from build123d import *

# Parameters (mm, degrees)
PAD026_DEPTH      = 10
SKETCH046_R       = 1.6
POCKET018_DEPTH   = 15.001
SKETCH047_R       = 4
POCKET019_DEPTH   = 2
POCKET019_FACE6_W = 8
POCKET019_FACE6_H = 20
POCKET024_DEPTH   = 6.1
CHAMFER008_SIZE   = 2
FILLET014_R       = 10
FILLET015_R       = 3
CHAMFER009_SIZE   = 1
SKETCH048_R       = 2.1
POCKET020_DEPTH   = 15.4865555595
CHAMFER010_SIZE   = 0.6


with BuildPart() as part:
    # Sketch045 → Pad026 (new body, symmetric)
    with BuildSketch(Plane.XY):
        Polygon((40, 50), (45, 50), (45, 38.2679491924), (37.9807621135, 34.2153903092), (43.3012701892, 25), (48.6217782649, 15.7846096908), (41.6935750346, 11.7846096908), (36.3730669589, 21), (30, 32.0384757729), (30, 40), (40, 40), align=None)
    extrude(amount=PAD026_DEPTH, both=True)

    # Sketch046 (on Face5 of Pad026) → Pocket018 (cut, through all)
    with BuildSketch(Plane.YZ.offset(45)):
        with Locations((45, 0)):
            Circle(SKETCH046_R)
    extrude(amount=-POCKET018_DEPTH, mode=Mode.SUBTRACT)

    # Sketch047 (on Face9 of Pocket018) → Pocket019 (cut)
    with BuildSketch(Plane.YZ.offset(45)):
        with Locations((45, 0)):
            Circle(SKETCH047_R)
    extrude(amount=-POCKET019_DEPTH, mode=Mode.SUBTRACT)

    # Pocket019 Face6 → Pocket024 (cut)
    with BuildSketch(Plane(origin=(45.1576766498, 13.7846096908, 0), x_dir=(-0.8660254038, -0.5, 0), z_dir=(0.5, -0.8660254038, 0))):
        Rectangle(POCKET019_FACE6_W, POCKET019_FACE6_H)
    extrude(amount=-POCKET024_DEPTH, mode=Mode.SUBTRACT)

    # Chamfer008
    chamfer008_edges = [part.edges().sort_by_distance(p)[0] for p in [
        (42.5, 50, 10),
        (42.5, 50, -10),
        (42.107677, 19.067365, 10),
        (42.107677, 19.067365, -10),
    ]]
    chamfer(chamfer008_edges, length=CHAMFER008_SIZE)

    # Fillet014
    fillet014_edges = [part.edges().sort_by_distance(p)[0] for p in [
        (30, 32.038476, 0),
    ]]
    fillet(fillet014_edges, radius=FILLET014_R)

    # Fillet015
    fillet015_edges = [part.edges().sort_by_distance(p)[0] for p in [
        (45, 38.267949, 0),
    ]]
    fillet(fillet015_edges, radius=FILLET015_R)

    # Chamfer009
    chamfer009_edges = [part.edges().sort_by_distance(p)[0] for p in [
        (30, 40, 0),
    ]]
    chamfer(chamfer009_edges, length=CHAMFER009_SIZE)

    # Sketch048 (on Face13 of Chamfer009) → Pocket020 (cut, through all)
    with BuildSketch(Plane(origin=(43.3012701892, 25, 0), x_dir=(-0.5, 0.8660254038, 0), z_dir=(0.8660254038, 0.5, 0))):
        Circle(SKETCH048_R)
    extrude(amount=-POCKET020_DEPTH, mode=Mode.SUBTRACT)

    # Chamfer010
    chamfer010_edges = [part.edges().sort_by_distance(p)[0] for p in [
        (44.35127, 23.181347, 0),
        (37.423067, 19.181347, 0),
    ]]
    chamfer(chamfer010_edges, length=CHAMFER010_SIZE)


with BuildPart() as part_1:
    # Body026 placement: moved
    add(part.part.moved(Location((0, 0, 56))))


solid = part_1.part
Verification items for the finished model (mm, model axes). A direction names the side the tool comes from. Coordinates: 2 decimals unless noted, no trailing zeros. Order: outer loops, then holes, each group sorted by start corner. A loop starts at its lowest first (then second) coordinate and runs counter-clockwise, first axis right, second up.
Item 1: Material ranges on L1, parallel to Z at x = 42.15, y = 45; L2, parallel to Z at x = 44.55, y = 45; L3, parallel to Y at x = 40.25, z = 55, recorded low to high.
Filled in:
L1: z = 46 to 54.4, 57.6 to 66
L2: z = 46 to 52, 60 to 66
L3: y = 17.99 to 21.11, 25.37 to 30.28, 35.53 to 43.75, 46.25 to 50
Item 2: Depth check by flat-ended pin: pin 1 (2 mm diameter, centred on y = 38, z = 56.5, fed in from +X); pin 2 (4 mm diameter, centred on x = 40.5, z = 63, fed in from -Y); pin 3 (6.5 mm diameter, centred on y = 46.5, z = 57, fed in from +X); pin 4 (1.9 mm diameter, centred on y = 45, z = 56, fed in from -X). Enter the tip coordinate at first touch or a pass-through.
Filled in:
pin 1: stops at x = 44.83
pin 2: stops at y = 17.07
pin 3: stops at x = 45
pin 4: passes through
Item 3: Section check A-A, the plane y = 45. Enter the section's corners in (x, z), then the cut area to 3 significant figures.
Filled in:
outline: (40, 46) - (45, 46) - (45, 52) - (43, 52) - (43, 54.4) - (40, 54.4) - close; (40, 57.6) - (43, 57.6) - (43, 60) - (45, 60) - (45, 66) - (40, 66) - close
area: 74.4 mm2
Item 4: Section check C-C, the plane x = 41. Give the number of separate pieces and of enclosed holes in the cut face, then the cut area to 3 significant figures.
Filled in:
separate pieces: 2
enclosed holes: 2
area: 459 mm2
Item 5: Access from +Z, -Z, +X, -X, +Y, -Y to the whole of each face (thin tool, end or side, straight path). Record for faces 1 (the face through (45, 48.4, 58.4)), 2 (the face through (40, 43, 56)), 3 (the face through (44.014, 44.133, 52.095)).
Filled in:
face 1: +Z, -Z, +X, +Y
face 2: +Z, -Z, -X, +Y
face 3: +X
Item 6: Release check for a two-part mould opening along Y. For faces 4 (the face through (42, 50, 56)), 5 (the face through (30, 37, 56)), 6 (the face through (41.83, 27.55, 56.14)) record: +Y half, -Y half, draft (parallel to the pull), parting line (faces both ways), or undercut.
Filled in:
face 4: +Y half
face 5: draft
face 6: undercut
Item 7: Section check B-B, the plane z = 62.5. Enter the section's corners in (x, y), then the cut area to 3 significant figures.
Filled in:
outline: (30, 34.72) arc R10 ccw to (31.34, 29.72) - (38.64, 17.07) - (45.57, 21.07) - (37.98, 34.22) - (43.5, 37.4) arc R3 ccw to (45, 40) - (45, 50) - (40, 50) - (40, 40) - (31, 40) - (30, 39) - close
area: 260 mm2
